Verification items for the finished model (mm, model axes). A direction names the side the tool comes from. Coordinates: 2 decimals unless noted, no trailing zeros. Write each loop counter-clockwise with the first axis right and the second up, starting at its lowest first coordinate (ties: lowest second). Pieces come first, ordered by that corner, then holes. Notation, with made-up numbers: M 56,75.25 L 91,75.25 A16 ccw 91,81.25 Z; hole C 20.25,-36 d4. An arc over 180 degrees is marked long. Answer in a Markdown table with one row per item.
from build123d import *

# Parameters (mm, degrees)
PAD_DEPTH    = 5
SKETCH001_W  = 5
SKETCH001_H  = 99.995
PAD001_DEPTH = 60
FILLET_R     = 2


with BuildPart() as part:
    # Sketch → Pad (new body)
    with BuildSketch(Plane.XY):
        with BuildLine():
            Line((0, 49.9975), (50, 49.9975))
            Line((50, 49.9975), (50, -49.9975))
            Line((50, -49.9975), (0, -49.9975))
            ThreePointArc((0, 49.9975), (-49.5, 0), (0, -49.9975))
        make_face()
    extrude(amount=PAD_DEPTH)

    # Sketch001 (on Face6 of Pad) → Pad001 (join)
    with BuildSketch(Plane.XY.offset(5)):
        with Locations((9.5, 0)):
            Rectangle(SKETCH001_W, SKETCH001_H)
        with Locations((42, 0)):
            Rectangle(SKETCH001_W, SKETCH001_H)
    extrude(amount=PAD001_DEPTH)

    # Fillet
    fillet_edges = [part.edges().sort_by_distance(p)[0] for p in [
        (50, 49.9975, 2.5),
        (50, -49.9975, 2.5),
        (50, 0, 0),
        (50, 0, 5),
        (25, 49.9975, 0),
        (25, -49.9975, 0),
        (-49.5, 0, 0),
        (0, 49.9975, 2.5),
        (0, -49.9975, 2.5),
        (-49.5, 0, 5),
        (3.5, 49.9975, 5),
        (7, 0, 5),
        (3.5, -49.9975, 5),
        (47.25, 49.9975, 5),
        (47.25, -49.9975, 5),
        (44.5, 0, 5),
        (7, 49.9975, 35),
        (7, -49.9975, 35),
        (7, 0, 65),
        (9.5, -49.9975, 65),
        (12, 0, 65),
        (9.5, 49.9975, 65),
        (25.75, 49.9975, 5),
        (39.5, 0, 5),
        (25.75, -49.9975, 5),
        (12, 0, 5),
        (12, -49.9975, 35),
        (12, 49.9975, 35),
        (39.5, 49.9975, 35),
        (39.5, -49.9975, 35),
        (39.5, 0, 65),
        (44.5, -49.9975, 35),
        (44.5, 49.9975, 35),
        (44.5, 0, 65),
        (42, -49.9975, 65),
        (42, 49.9975, 65),
    ]]
    fillet(fillet_edges, radius=FILLET_R)


solid = part.part
1) Tool access check on faces 1 (the face through (44.5, -1, 35)), 2 (the face through (9.7, 49.998, 23.3)), 3 (the face through (39.5, -1, 35)), 4 (the face through (-15, 1, 5)). Record the directions out of +Z, -Z, +X, -X, +Y, -Y that give a thin tool (end or side, any length) a straight path to the whole face; none if there is none.
Response values:
| item | result |
|---|---|
| face 1 | +Z, +X, +Y, -Y |
| face 2 | +Z, -Z, +X, -X, +Y |
| face 3 | +Z, +Y, -Y |
| face 4 | +Z, -X, +Y, -Y |
2) Sectioned sample at C-C (y = 0). Record the cut outline in (x, z).
Response values:
| item | result |
|---|---|
| outline | M -49.5,2 A2 ccw -47.5,0 L 48,0 A2 ccw 50,2 L 50,3 A2 ccw 48,5 L 46.5,5 A2 cw 44.5,7 L 44.5,63 A2 ccw 42.5,65 L 41.5,65 A2 ccw 39.5,63 L 39.5,7 A2 cw 37.5,5 L 14,5 A2 cw 12,7 L 12,63 A2 ccw 10,65 L 9,65 A2 ccw 7,63 L 7,7 A2 cw 5,5 L -47.5,5 A2 ccw -49.5,3 Z |
3) Depth check by flat-ended pin: pin 1 (1.2 mm diameter, centred on x = 47, y = 14, fed in from +Z); pin 2 (6 mm diameter, centred on x = 5.5, y = -17.5, fed in from +Z); pin 3 (17 mm diameter, centred on y = -3.5, z = 43, fed in from +X). Enter the tip coordinate at first touch or a pass-through.
Response values:
| item | result |
|---|---|
| pin 1 | stops at z = 5 |
| pin 2 | stops at z = 64.94 |
| pin 3 | stops at x = 44.5 |
4) Sectioned sample at B-B (x = 16.5). Record the cut outline in (y, z).
Response values:
| item | result |
|---|---|
| outline | M -50,2 A2 ccw -48,0 L 48,0 A2 ccw 50,2 L 50,3 A2 ccw 48,5 L -48,5 A2 ccw -50,3 Z |
5) Sectioned sample at A-A (z = 40). Record the cut outline in (x, y), then the cut area to 3 significant figures.
Response values:
| item | result |
|---|---|
| outline | M 7,-48 A2 ccw 9,-50 L 10,-50 A2 ccw 12,-48 L 12,48 A2 ccw 10,50 L 9,50 A2 ccw 7,48 Z; M 39.5,-48 A2 ccw 41.5,-50 L 42.5,-50 A2 ccw 44.5,-48 L 44.5,48 A2 ccw 42.5,50 L 41.5,50 A2 ccw 39.5,48 Z |
| area | 993 mm² |
6) Thickness scan on L1, parallel to X at y = 3, z = 55; L2, parallel to Z at x = -18, y = 26.5; L3, parallel to Y at x = 10.5, z = 11. Record the ranges inside material, lowest first. Write a range as [from, to].
Response values:
| item | result |
|---|---|
| L1 | x = [7, 12], [39.5, 44.5] |
| L2 | z = [0, 5] |
| L3 | y = [-49.93, 49.93] |
